Here's the drawing with two shaded views (mm, measured from the low corner). I have some questions. Give positions to 0.01 mm unless a question says otherwise; leave off trailing zeros. Loops run counter-clockwise (first coordinate to the right, second up) from the corner with the lowest first, then second, coordinate; pieces in that order, holes last. Notation, with made-up numbers: M 2,5 L 12,5 A18 cw 12,39 Z; hole C 58,68.5 d11. An arc over 180 degrees is marked long. Use a Markdown table: item, result. Add a question column.
1) Will these pins go through, and if not, where does the flat tip stop? pin 1 Ø2 at (x, y) = (18.5, 1) entering from -Z; pin 2 Ø6 at (x, z) = (33.5, 35.5) entering from -Y.
2) Suppose I cut it at A-A on z = 15. List the corners of the cut face in (x, y) for me.
3) Suppose I cut it at C-C on y = 4.75. Count the separate pieces of the cut face and the enclosed holes in it, and give its area (3 significant figures).
4) We'd pull the mould along Z, two halves only. Please class the marked faces 1, 2 and 3: +Z half, -Z half, draft (parallel to the pull), parting line (faces both ways), or undercut.
5) If I drill on line 1 along X through (y, z) = (2.75, 24) (1 decimal); line 2 along X through (y, z) = (4.5, 45) (1 decimal); line 3 along X through (y, z) = (1.25, 15.5) (1 decimal), over which ranges is the centre line in solid material (lowest first)? Write a range as [from, to].
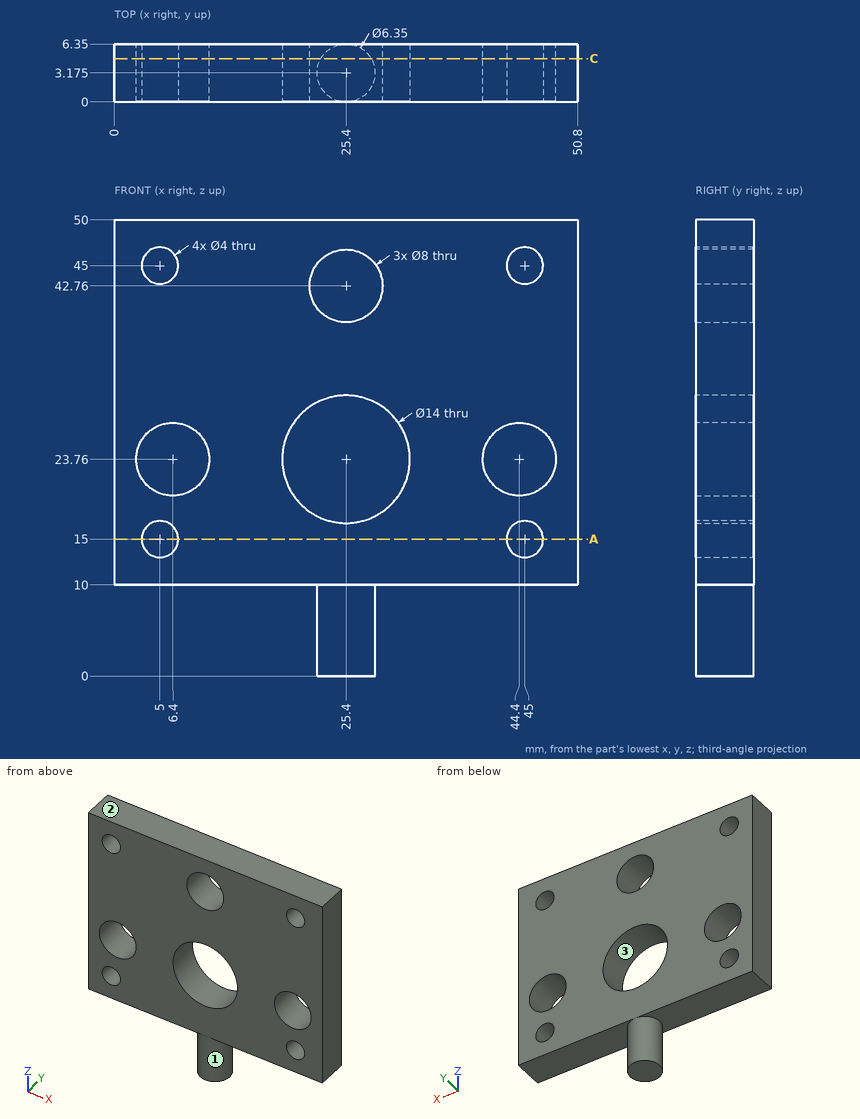
Answer block:
| question | item | result |
|---|---|---|
| 1 | pin 1 | stops at z = 10 |
| 1 | pin 2 | stops at y = 0 |
| 2 | outline | M 0,0 L 3,0 L 3,6.35 L 0,6.35 Z; M 7,0 L 43,0 L 43,6.35 L 7,6.35 Z; M 47,0 L 50.8,0 L 50.8,6.35 L 47,6.35 Z |
| 3 | separate pieces | 1 |
| 3 | enclosed holes | 8 |
| 3 | area | 1,730 mm^2 |
| 4 | face 1 | draft |
| 4 | face 2 | +Z half |
| 4 | face 3 | undercut |
| 5 | line 1 | x = [0, 2.4], [10.4, 18.4], [32.4, 40.4], [48.4, 50.8] |
| 5 | line 2 | x = [0, 3], [7, 22.1], [28.7, 43], [47, 50.8] |
| 5 | line 3 | x = [0, 3.1], [6.9, 43.1], [46.9, 50.8] |
